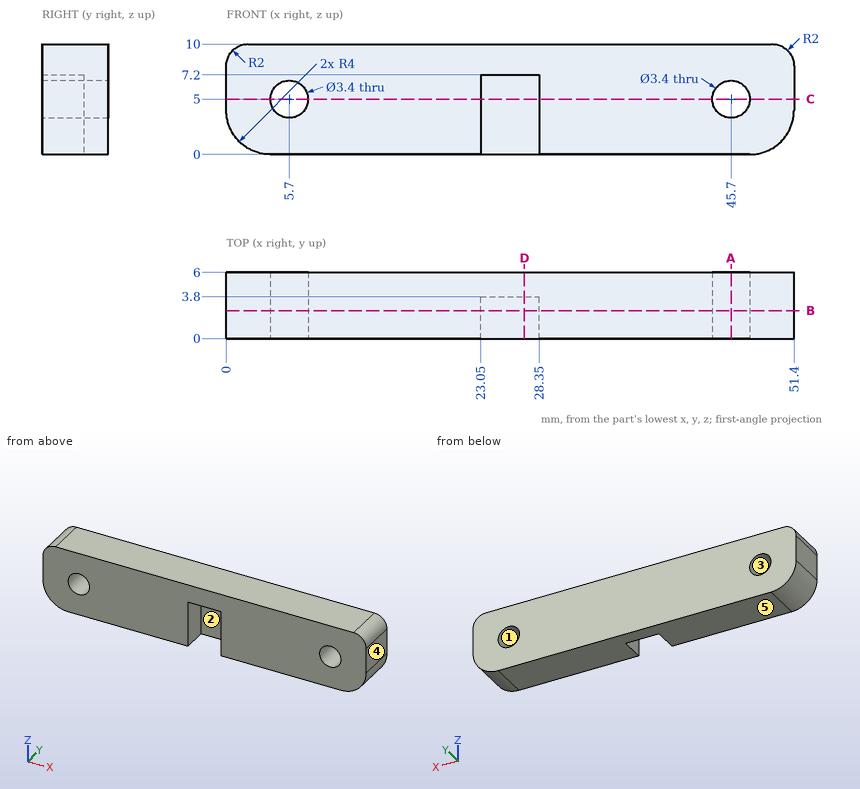
Study the drawing (mm; zero at the part's minimum x, y, z) and answer. A direction names the side the tool comes from. Give positions to 0.01 mm unless a question says otherwise; leave off trailing zeros. Write each loop counter-clockwise with the first axis right and the second up, starting at its lowest first coordinate (ties: lowest second). Pieces come first, ordered by that corner, then holes. Notation, with made-up numbers: (32.25, 48.25) -> (51.25, 48.25) arc R22 ccw to (51.25, 86.25) -> close; hole circle Ø5 at (59, -29). An arc over 180 degrees is marked (long way). Answer in a Markdown table with one row per item.
1) Straight lines are drawn through the part: line 1 (X direction, y = 4.2, z = 5); line 2 (X direction, y = 3.1, z = 5); line 3 (X direction, y = 3.25, z = 4). For each, find the intervals that lie inside material, in ascending order. Write a range as [from, to].
Results list:
| item | result |
|---|---|
| line 1 | [0, 4], [7.4, 44], [47.4, 51.4] |
| line 2 | [0, 4], [7.4, 23.05], [28.35, 44], [47.4, 51.4] |
| line 3 | [0, 4.33], [7.07, 23.05], [28.35, 44.33], [47.07, 51.4] |
2) Each of these flat-tipped pins is pushed along its axis until it touches: pin 1 Ø1.9 at (x, y) = (25, 2) entering from -Z; pin 2 Ø1.9 at (y, z) = (2.5, 2) entering from -X. Where does it stop, or does it pass through?
Results list:
| item | result |
|---|---|
| pin 1 | z = 7.2 |
| pin 2 | x = 0.14 |
3) A tool of negligible diameter and unlimited length cuts with its end or side. For the marked faces 1 and 2, from which of +Z, -Z, +X, -X, +Y, -Y can it reach the whole face along a straight path? Write none if from no direction.
Results list:
| item | result |
|---|---|
| face 1 | +Y, -Y |
| face 2 | -Z, -Y |
4) Section A-A on x = 45.7 is taken. Give the vertices of the cut face in (y, z).
Results list:
| item | result |
|---|---|
| outline | (0, 0) -> (6, 0) -> (6, 3.3) -> (0, 3.3) -> close; (0, 6.7) -> (6, 6.7) -> (6, 10) -> (0, 10) -> close |
5) Section C-C on z = 5 is taken. Give the vertices of the cut face in (x, y), plus the area to 3 significant figures.
Results list:
| item | result |
|---|---|
| outline | (0, 0) -> (4, 0) -> (4, 6) -> (0, 6) -> close; (7.4, 0) -> (23.05, 0) -> (23.05, 3.8) -> (28.35, 3.8) -> (28.35, 0) -> (44, 0) -> (44, 6) -> (7.4, 6) -> close; (47.4, 0) -> (51.4, 0) -> (51.4, 6) -> (47.4, 6) -> close |
| area | 247 mm^2 |
6) Section D-D on x = 27 is taken. Give the vertices of the cut face in (y, z).
Results list:
| item | result |
|---|---|
| outline | (0, 7.2) -> (3.8, 7.2) -> (3.8, 0) -> (6, 0) -> (6, 10) -> (0, 10) -> close |
7) Determine the mould class of the marked faces 3, 4 and 5 for opening direction Z: released by +Z, released by -Z, zero draft, split by the parting line, or undercut.
Results list:
| item | result |
|---|---|
| face 3 | undercut |
| face 4 | zero draft |
| face 5 | released by -Z |
8) Section B-B on y = 2.55 is taken. Give the vertices of the cut face in (x, z).
Results list:
| item | result |
|---|---|
| outline | (0, 4) arc R4 ccw to (4, 0) -> (23.05, 0) -> (23.05, 7.2) -> (28.35, 7.2) -> (28.35, 0) -> (47.4, 0) arc R4 ccw to (51.4, 4) -> (51.4, 8) arc R2 ccw to (49.4, 10) -> (2, 10) arc R2 ccw to (0, 8) -> close; hole circle Ø3.4 at (5.7, 5); hole circle Ø3.4 at (45.7, 5) |
